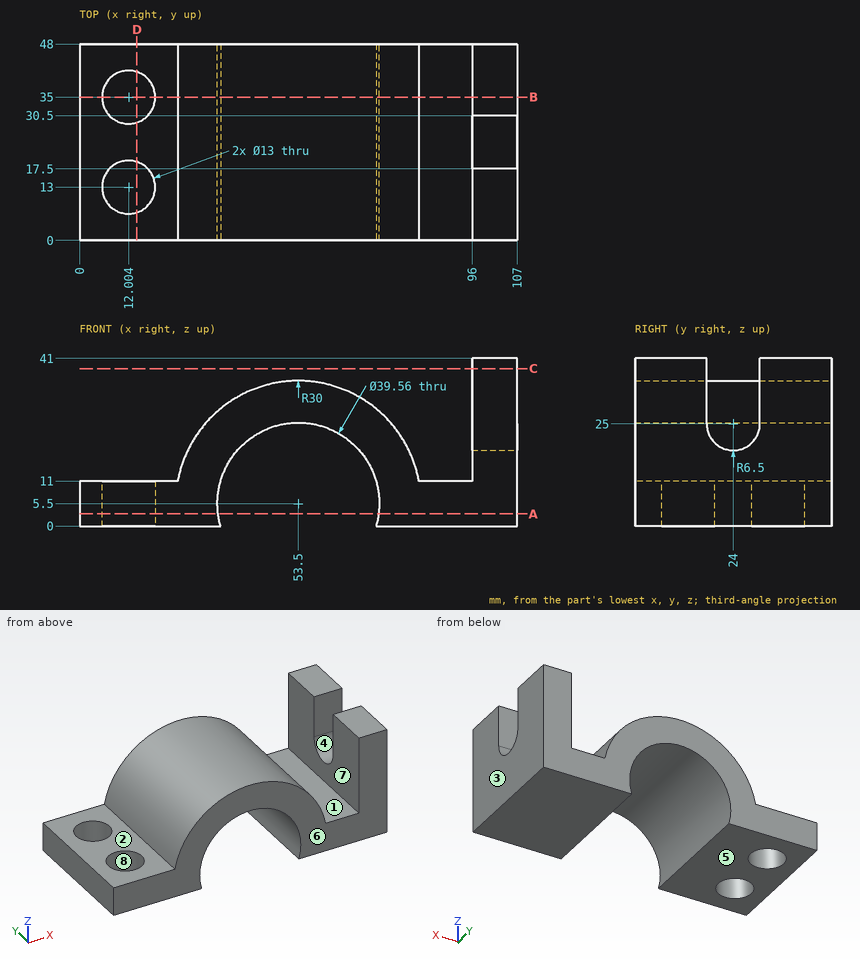
Could you check a few things on this drawing? It's one solid part, dimensions in mm from its lowest x, y, z. A direction names the side the tool comes from. Give positions to 0.01 mm unless a question says otherwise; leave off trailing zeros. Loops run counter-clockwise (first coordinate to the right, second up) from the corner with the lowest first, then second, coordinate; pieces in that order, holes last. Notation, with made-up numbers: M 3.5,82.5 L 29.5,82.5 A12 cw 29.5,88.5 Z; hole C 43.25,45 d2. An arc over 180 degrees is marked long. One line per question, with ' | ' between items. Start each with the question number.
Q1. If I drill on line 1 (X direction, y = 32, z = 5); line 2 (X direction, y = 21, z = 5.5); line 3 (Y direction, x = 17.5, z = 2.5), over which ranges is the centre line in solid material (lowest first)? Write a range as from..to.
Q2. For the marked faces 1, 2, 3, 4 and 5, which set-ups out of +Z, -Z, +X, -X, +Y, -Y let a thin tool reach every point of the face, with its end or its side?
Q3. If we section it at B-B (y = 35): Please give me the cut outline in (x, z), plus the area to 3 significant figures.
Q4. If we section it at A-A (z = 3): Please give me the cut outline in (x, y).
Q5. If we mould it in two halves opening along Y, with no side actions, what happens to the marked faces 6, 7 and 8? For each: +Y half, -Y half, draft (parallel to the pull), parting line (faces both ways), or undercut.
Q6. If we section it at D-D (x = 14): Please give me the cut outline in (y, z).
Q7. If we section it at C-C (z = 38.5): Please give me the cut outline in (x, y), plus the area to 3 significant figures.
Q8. For pin 1 Ø1 at (y, z) = (41.5, 27.5) entering from -X; pin 2 Ø12 at (x, z) = (53.5, 15.5) entering from -Y; pin 3 Ø2 at (x, y) = (41, 40) entering from +Z; pin 4 Ø15 at (y, z) = (15.5, 30) entering from -X, each with a flat end and sliding along its axis, tell me the tip position at first contact or that it passes through.
Computed:
1) line 1: x = 0..6.24, 17.77..33.73, 73.27..107 | line 2: x = 0..33.72, 73.28..107 | line 3: y = 0..9.53, 16.47..31.53, 38.47..48
2) face 1: +Z, +Y, -Y | face 2: +Z, -X, +Y, -Y | face 3: +Z, -Z, +X, +Y, -Y | face 4: +Z, +X | face 5: -Z, +X, -X, +Y, -Y
3) outline: M 0,0 L 5.5,0 L 5.5,11 L 0,11 Z; M 18.5,0 L 34.5,0 A19.78 cw long 72.5,0 L 107,0 L 107,41 L 96,41 L 96,11 L 82.99,11 A30 ccw 24.01,11 L 18.5,11 Z | area: 1,620 mm²
4) outline: M 0,0 L 33.88,0 L 33.88,48 L 0,48 Z; M 73.12,0 L 107,0 L 107,48 L 73.12,48 Z; hole C 12,13 d13; hole C 12,35 d13
5) face 6: -Y half | face 7: draft | face 8: undercut
6) outline: M 0,0 L 6.81,0 L 6.81,11 L 0,11 Z; M 19.19,0 L 28.81,0 L 28.81,11 L 19.19,11 Z; M 41.19,0 L 48,0 L 48,11 L 41.19,11 Z
7) outline: M 96,0 L 107,0 L 107,17.5 L 96,17.5 Z; M 96,30.5 L 107,30.5 L 107,48 L 96,48 Z | area: 385 mm²
8) pin 1: stops at x = 32.58 | pin 2: passes through | pin 3: stops at z = 33.21 | pin 4: stops at x = 28.78
